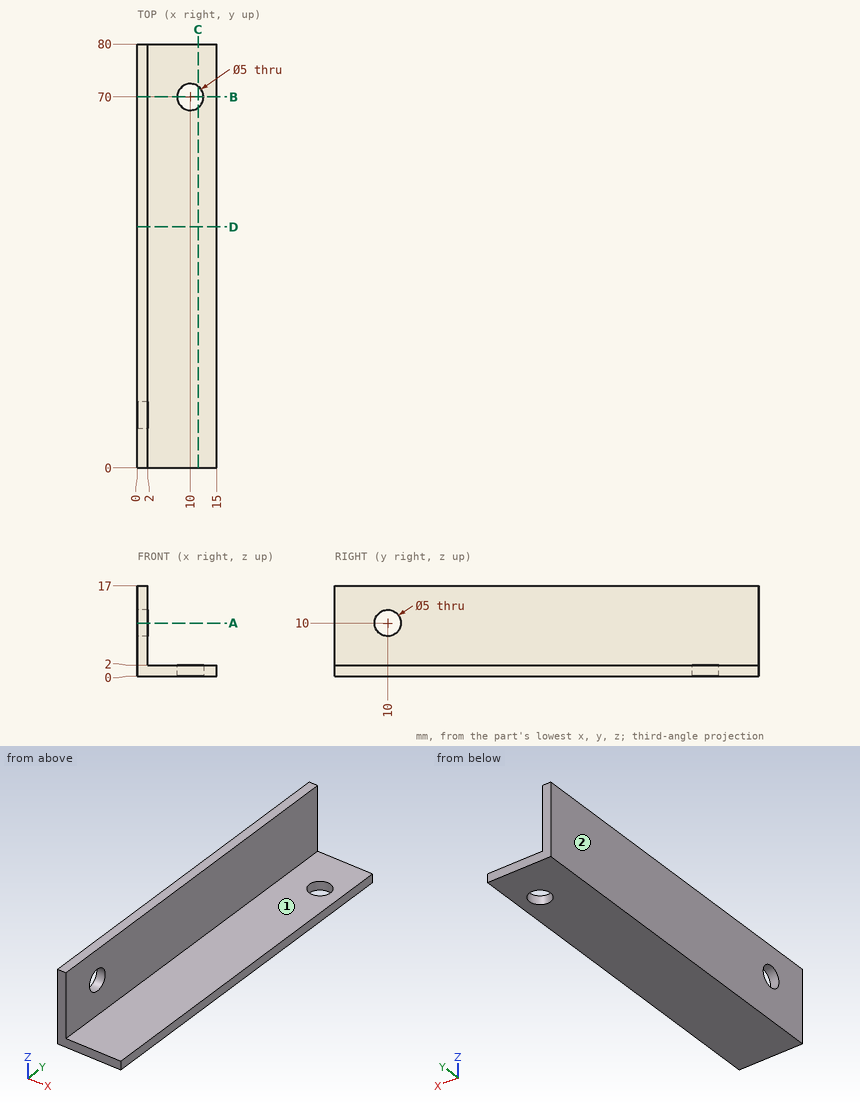
Could you check a few things on this drawing? It's one solid part, dimensions in mm from its lowest x, y, z. A direction names the side the tool comes from. Coordinates: 2 decimals unless noted, no trailing zeros. Order: outer loops, then holes, each group sorted by start corner. A loop starts at its lowest first (then second) coordinate and runs counter-clockwise, first axis right, second up. Notation, with made-up numbers: M -15.75,7.25 L 40.25,7.25 A24 cw 40.25,41.25 Z; hole C 1,40 d1. An arc over 180 degrees is marked long. Answer as a JSON object with one key per item and string values. Group by question number.
(1) I need wall thicknesses on probe 1 along Z at (x, y) = (1.5, 10); probe 2 along Y at (x, z) = (1, 10.25); probe 3 along Y at (x, z) = (10, 0.9). Which ranges of each line are inside material? Lowest first, please.
(2) Suppose I cut it at D-D, the plane y = 45.5. Please give me the cut outline in (x, z).
(3) Suppose I cut it at C-C, the plane x = 11.5. Please give me the cut outline in (y, z).
(4) Which directions (+Z, -Z, +X, -X, +Y, -Y) give clear straight access to the entire face, cutting with the end or side of a thin tool? Please do the marked faces 1 and 2.
(5) Suppose I cut it at A-A, the plane z = 10. Please give me the cut outline in (x, y).
(6) For pin 1 (1 mm diameter, centred on x = 10, y = 57, fed in from -Z); pin 2 (2 mm diameter, centred on y = 9.5, z = 15, fed in from +X); pin 3 (4 mm diameter, centred on x = 8.5, y = 30.5, fed in from +Z), each with a flat end and sliding along its axis, tell me the tip position at first contact or that it passes through.
(7) Suppose I cut it at B-B, the plane y = 70. Please give me the cut outline in (x, z), then the cut area to 3 significant figures.
Values found:
{
 "1": {"probe 1": "z = 0 to 7.5, 12.5 to 17", "probe 2": "y = 0 to 7.51, 12.49 to 80", "probe 3": "y = 0 to 67.5, 72.5 to 80"},
 "2": {"outline": "M 0,0 L 15,0 L 15,2 L 2,2 L 2,17 L 0,17 Z"},
 "3": {"outline": "M 0,0 L 68,0 L 68,2 L 0,2 Z; M 72,0 L 80,0 L 80,2 L 72,2 Z"},
 "4": {"face 1": "+Z, +X, +Y, -Y", "face 2": "+Z, -Z, -X, +Y, -Y"},
 "5": {"outline": "M 0,0 L 2,0 L 2,7.5 L 0,7.5 Z; M 0,12.5 L 2,12.5 L 2,80 L 0,80 Z"},
 "6": {"pin 1": "stops at z = 0", "pin 2": "stops at x = 2", "pin 3": "stops at z = 2"},
 "7": {"outline": "M 0,0 L 7.5,0 L 7.5,2 L 2,2 L 2,17 L 0,17 Z; M 12.5,0 L 15,0 L 15,2 L 12.5,2 Z", "area": "50.0 mm^2"}
}
